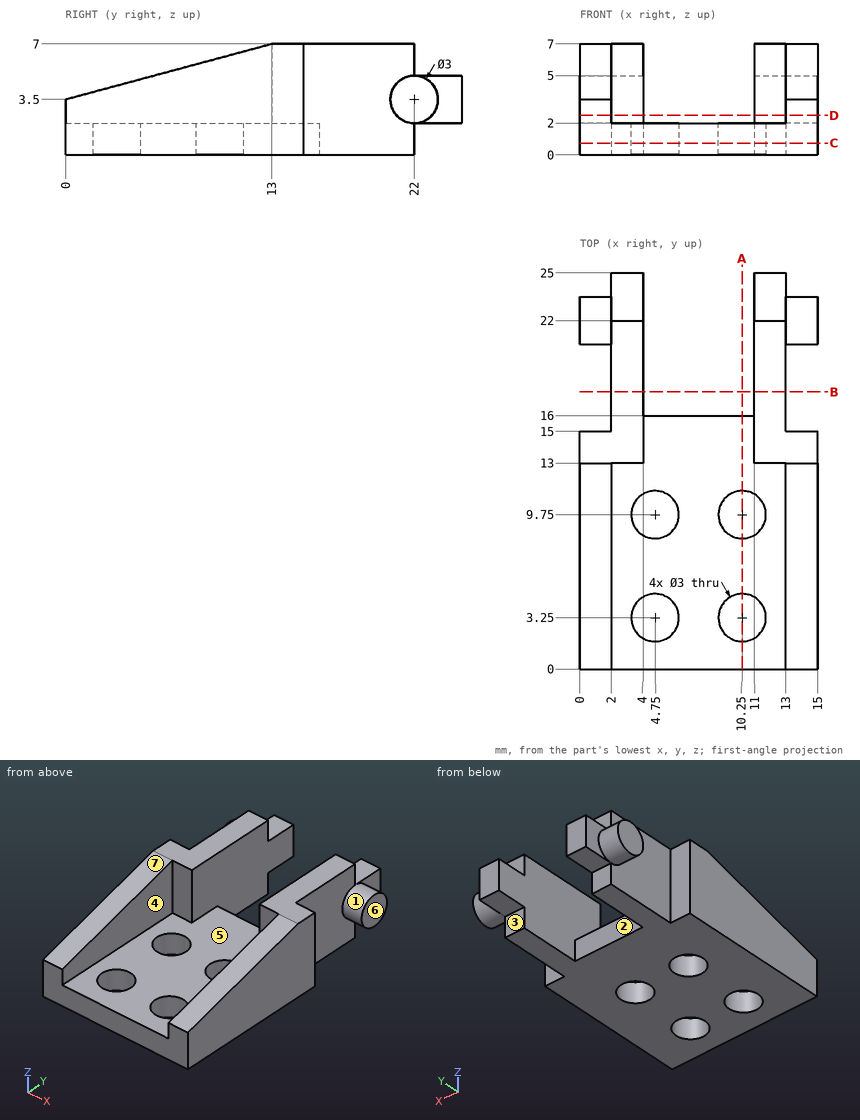
Drawing for the job (mm, zero at the part's lowest x, y, z). A direction names the side the tool comes from. Round coordinates to 2 decimals unless told otherwise and drop trailing zeros. Order: outer loops, then holes, each group sorted by start corner. A loop starts at its lowest first (then second) coordinate and runs counter-clockwise, first axis right, second up.
Item 1: Saw through at B-B on y = 17.5. Write the cut outline in (x, z), then the cut area to 3 significant figures.
Item 2: Saw through at C-C on z = 0.75. Write the cut outline in (x, y), then the cut area to 3 significant figures.
Item 3: Probe line 1 along Y through (x, z) = (4.75, 1.3); line 2 along X through (y, z) = (8, 3); line 3 along X through (y, z) = (18.25, 4.25). List the from-to ranges inside material, lowest first.
Item 4: Saw through at A-A on x = 10.25. Write the cut outline in (y, z).
Item 5: Mould opens along X. For the marked faces 5, 6 and 7 say: pulls with the +X half, pulls with the -X half, needs draft (parallel to the pull), parting line crosses it, or undercut.
Item 6: Saw through at D-D on z = 2.5. Write the cut outline in (x, y), then the cut area to 3 significant figures.
Item 7: Pin check, flat tips, straight feed: pin 1 (1 mm diameter, centred on x = 6, y = 20, fed in from -Z); pin 2 (0.6 mm diameter, centred on x = 12.5, z = 1, fed in from +Y); pin 3 (1 mm diameter, centred on x = 12.5, y = 23, fed in from -Z); pin 4 (5.5 mm diameter, centred on x = 9.5, y = 10, fed in from +Z). Stop position of each tip, or through.
Item 8: Tool access for the marked faces 1, 2, 3 and 4: list every direction of +Z, -Z, +X, -X, +Y, -Y with a clear straight run to the whole face (end or side of a thin tool).
Reported:
1. outline: (2, 0) - (4, 0) - (4, 7) - (2, 7) - close; (11, 0) - (13, 0) - (13, 7) - (11, 7) - close
1. area: 28.0 mm2
2. outline: (0, 0) - (15, 0) - (15, 15) - (13, 15) - (13, 22) - (11, 22) - (11, 16) - (4, 16) - (4, 22) - (2, 22) - (2, 15) - (0, 15) - close; hole circle Ø3 at (4.75, 3.25); hole circle Ø3 at (4.75, 9.75); hole circle Ø3 at (10.25, 3.25); hole circle Ø3 at (10.25, 9.75)
2. area: 232 mm2
3. line 1: y = 0 to 1.75, 4.75 to 8.25, 11.25 to 16
3. line 2: x = 0 to 2, 13 to 15
3. line 3: x = 2 to 4, 11 to 13
4. outline: (0, 0) - (1.75, 0) - (1.75, 2) - (0, 2) - close; (4.75, 0) - (8.25, 0) - (8.25, 2) - (4.75, 2) - close; (11.25, 0) - (16, 0) - (16, 2) - (11.25, 2) - close
5. face 5: undercut
5. face 6: pulls with the +X half
5. face 7: needs draft
6. outline: (0, 0) - (2, 0) - (2, 13) - (4, 13) - (4, 25) - (2, 25) - (2, 23.12) - (0, 23.12) - (0, 20.88) - (2, 20.88) - (2, 15) - (0, 15) - close; (11, 13) - (13, 13) - (13, 0) - (15, 0) - (15, 15) - (13, 15) - (13, 20.88) - (15, 20.88) - (15, 23.12) - (13, 23.12) - (13, 25) - (11, 25) - close
6. area: 117 mm2
7. pin 1: passes through
7. pin 2: stops at y = 22
7. pin 3: stops at z = 2
7. pin 4: stops at z = 2
8. face 1: +X
8. face 2: +Z, -Z, +Y
8. face 3: -Z, +X, -X, +Y
8. face 4: +Z, -Y
